```python
from build123d import *

# Parameters (mm, degrees)
BOSS_EXTRUDE1_DEPTH = 20
SKETCH2_R           = 37.5
BOSS_EXTRUDE2_DEPTH = 40
CUT_EXTRUDE1_REACH  = 148.969
SKETCH3_R           = 2.5
SKETCH4_R           = 27.5
CUT_EXTRUDE2_DEPTH  = 154.622914957


with BuildPart() as part:
    # Sketch1 → Boss-Extrude1 (new body)
    with BuildSketch(Plane(origin=(0, 0, 0), x_dir=(1, 0, 0), z_dir=(0, 1, 0))):
        with BuildLine():
            Line((-90, -100), (90, -100))
            ThreePointArc((90, -100), (97.071067812, -97.071067812), (100, -90))
            Line((100, -90), (100, 90))
            ThreePointArc((100, 90), (97.071067812, 97.071067812), (90, 100))
            Line((90, 100), (-90, 100))
            ThreePointArc((-90, 100), (-97.071067812, 97.071067812), (-100, 90))
            Line((-100, 90), (-100, -90))
            ThreePointArc((-100, -90), (-97.071067812, -97.071067812), (-90, -100))
        make_face()
    extrude(amount=BOSS_EXTRUDE1_DEPTH)

    # Sketch2 → Boss-Extrude2 (add)
    with BuildSketch(Plane(origin=(0, 20, 0), x_dir=(1, 0, 0), z_dir=(0, 1, 0))):
        with Locations(Location((0, 0, 0), (0, 0, 270))):
            Circle(SKETCH2_R)
    extrude(amount=BOSS_EXTRUDE2_DEPTH)

    # Sketch3 → Cut-Extrude1 (cut, up to next)
    with BuildSketch(Plane(origin=(0, 20, 0), x_dir=(1, 0, 0), z_dir=(0, 1, 0)), mode=Mode.PRIVATE) as cut_extrude1_sk1:
        with Locations(Location((-80, 80, 0), (0, 0, 270))):
            Circle(SKETCH3_R)
    cut_extrude1_tool1 = extrude(cut_extrude1_sk1.sketch, amount=-CUT_EXTRUDE1_REACH, mode=Mode.PRIVATE) & part.part
    # Sketch3 → Cut-Extrude1 (cut, up to next)
    with BuildSketch(Plane(origin=(0, 20, 0), x_dir=(1, 0, 0), z_dir=(0, 1, 0)), mode=Mode.PRIVATE) as cut_extrude1_sk2:
        with Locations(Location((80, 80, 0), (0, 0, 270))):
            Circle(SKETCH3_R)
    cut_extrude1_tool2 = extrude(cut_extrude1_sk2.sketch, amount=-CUT_EXTRUDE1_REACH, mode=Mode.PRIVATE) & part.part
    # Sketch3 → Cut-Extrude1 (cut, up to next)
    with BuildSketch(Plane(origin=(0, 20, 0), x_dir=(1, 0, 0), z_dir=(0, 1, 0)), mode=Mode.PRIVATE) as cut_extrude1_sk3:
        with Locations(Location((80, -80, 0), (0, 0, 270))):
            Circle(SKETCH3_R)
    cut_extrude1_tool3 = extrude(cut_extrude1_sk3.sketch, amount=-CUT_EXTRUDE1_REACH, mode=Mode.PRIVATE) & part.part
    # Sketch3 → Cut-Extrude1 (cut, up to next)
    with BuildSketch(Plane(origin=(0, 20, 0), x_dir=(1, 0, 0), z_dir=(0, 1, 0)), mode=Mode.PRIVATE) as cut_extrude1_sk4:
        with Locations(Location((-80, -80, 0), (0, 0, 270))):
            Circle(SKETCH3_R)
    cut_extrude1_tool4 = extrude(cut_extrude1_sk4.sketch, amount=-CUT_EXTRUDE1_REACH, mode=Mode.PRIVATE) & part.part
    add(cut_extrude1_tool1.solids().sort_by_distance((-80, 20, -80))[0], mode=Mode.SUBTRACT)
    add(cut_extrude1_tool2.solids().sort_by_distance((80, 20, -80))[0], mode=Mode.SUBTRACT)
    add(cut_extrude1_tool3.solids().sort_by_distance((80, 20, 80))[0], mode=Mode.SUBTRACT)
    add(cut_extrude1_tool4.solids().sort_by_distance((-80, 20, 80))[0], mode=Mode.SUBTRACT)

    # Sketch4 → Cut-Extrude2 (cut, through all)
    with BuildSketch(Plane(origin=(0, 60, 0), x_dir=(1, 0, 0), z_dir=(0, 1, 0))):
        with Locations(Location((0, 0, 0), (0, 0, 270))):
            Circle(SKETCH4_R)
    extrude(amount=-CUT_EXTRUDE2_DEPTH, mode=Mode.SUBTRACT)


solid = part.part
```
CAD build for the part. Positions are in the model's coordinates, mm. A direction names the side the tool comes from. Round coordinates to 2 decimals unless told otherwise and drop trailing zeros. Order: outer loops, then holes, each group sorted by start corner. A loop starts at its lowest first (then second) coordinate and runs counter-clockwise, first axis right, second up. Notation, with made-up numbers: (4.25, 85) - (19.25, 85) arc R13 cw to (19.25, 109) - close; hole circle Ø3 at (44.5, 17.5). An arc over 180 degrees is marked (long way). Answer as CSV lines item,"result". Start each with the question number.
1. Saw through at B-B, the plane z = 80. Write the cut outline in (x, y), and give its area (3 significant figures).
2. Saw through at A-A, the plane x = -80. Write the cut outline in (y, z), and give its area (3 significant figures).
3. Saw through at C-C, the plane z = 6.5. Write the cut outline in (x, y), and give its area (3 significant figures).
4. Saw through at D-D, the plane y = 50. Write the cut outline in (x, z), and give its area (3 significant figures).
5. Drill centre lines: L1, parallel to X at y = 10, z = 80; L2, parallel to X at y = 18, z = 0; L3, parallel to Y at x = -50.5, z = 43. Where is each one in solid material? Low to high. Write a range as [from, to].
6. Tool access for faces 5 (the face through (96.99, 9.86, 97.15)), 6 (the face through (-1, 20, -46)): list every direction of +Z, -Z, +X, -X, +Y, -Y with a clear straight run to the whole face (end or side of a thin tool).
7. Pull direction Z, two halves, no side cores. Call faces 1 (the face through (-79.9, 10.1, -82.5)), 2 (the face through (1, 10, -100)), 3 (the face through (-22.818, 39.72, -29.759)), 4 (the face through (80.1, 10.1, -82.5)): +Z half, -Z half, draft (parallel to the pull), parting line (faces both ways), or undercut.
8. Pin check, flat tips, straight feed: pin 1 (4 mm diameter, centred on y = 26, z = 27, fed in from +X); pin 2 (6.5 mm diameter, centred on x = 80, z = -80, fed in from +Y); pin 3 (3 mm diameter, centred on x = -80, z = 80, fed in from +Y); pin 4 (5 mm diameter, centred on x = -5.5, y = 46, fed in from +Z). Stop position of each tip, or through.
Model answer:
1,outline,"(-100, 0) - (-82.5, 0) - (-82.5, 20) - (-100, 20) - close; (-77.5, 0) - (77.5, 0) - (77.5, 20) - (-77.5, 20) - close; (82.5, 0) - (100, 0) - (100, 20) - (82.5, 20) - close"
1,area,"3,800 mm²"
2,outline,"(0, -100) - (20, -100) - (20, -82.5) - (0, -82.5) - close; (0, -77.5) - (20, -77.5) - (20, 77.5) - (0, 77.5) - close; (0, 82.5) - (20, 82.5) - (20, 100) - (0, 100) - close"
2,area,"3,800 mm²"
3,outline,"(-100, 0) - (-26.72, 0) - (-26.72, 60) - (-36.93, 60) - (-36.93, 20) - (-100, 20) - close; (26.72, 0) - (100, 0) - (100, 20) - (36.93, 20) - (36.93, 60) - (26.72, 60) - close"
3,area,"3,750 mm²"
4,outline,"circle Ø75 at (0, 0); hole circle Ø55 at (0, 0)"
4,area,"2,040 mm²"
5,L1,"x = [-100, -82.5], [-77.5, 77.5], [82.5, 100]"
5,L2,"x = [-100, -27.5], [27.5, 100]"
5,L3,"y = [0, 20]"
6,face 5,"+Z, +X, +Y, -Y"
6,face 6,"+Y"
7,face 1,"undercut"
7,face 2,"-Z half"
7,face 3,"parting line"
7,face 4,"undercut"
8,pin 1,"stops at x = 27.95"
8,pin 2,"stops at y = 20"
8,pin 3,"passes through"
8,pin 4,"stops at z = 37.38"
